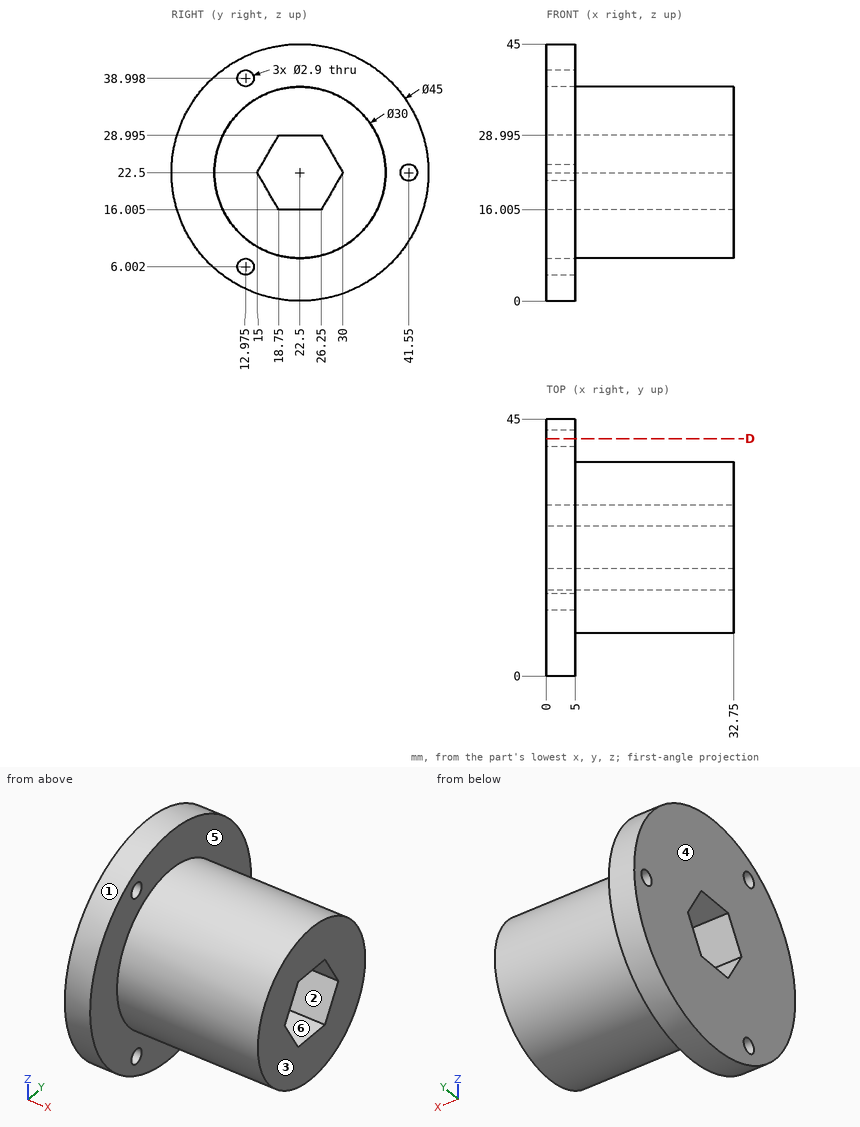
The figure shows three views and two pictorial views of one solid part (mm, origin at its lowest corner). Answer the questions. A direction names the side the tool comes from. Round coordinates to 2 decimals unless told otherwise and drop trailing zeros. Order: outer loops, then holes, each group sorted by start corner. A loop starts at its lowest first (then second) coordinate and runs counter-clockwise, first axis right, second up.
Q1. Find the intervals of material crossed by line 1 along Y through (x, z) = (2.2, 22.5); line 2 along Y through (x, z) = (1, 22) (1 decimal); line 3 along X through (y, z) = (43, 28), in increasing order.
Solution:
line 1: y = 0 to 15, 30 to 40.1, 43 to 45
line 2: y = 0 to 15.3, 29.7 to 40.2, 42.9 to 45
line 3: x = 0 to 5
Q2. The mould has two halves that part along Y. Classify the marked faces 1, 2 and 3: pulls with the +Y half, pulls with the -Y half, needs draft (parallel to the pull), parting line crosses it, or undercut.
Solution:
face 1: parting line crosses it
face 2: undercut
face 3: needs draft
Q3. A tool of negligible diameter and unlimited length cuts with its end or side. For the marked faces 4, 5 and 6, from which of +Z, -Z, +X, -X, +Y, -Y can it reach the whole face along a straight path? Write none if from no direction.
Solution:
face 4: +Z, -Z, -X, +Y, -Y
face 5: +X
face 6: +X, -X
Q4. Given pin 1 Ø1 at (x, z) = (29, 11) entering from +Y; pin 2 Ø6 at (x, y) = (18, 22) entering from -Z; pin 3 Ø1.5 at (x, y) = (16, 33.5) entering from -Z, each flat-ended and moving along its own axis, determine where each tip first touches the part or whether it passes through.
Solution:
pin 1: stops at y = 32.7
pin 2: stops at z = 7.5
pin 3: stops at z = 11.55
Q5. A cutting plane is placed at D-D, the plane y = 41.55. Determine the outline of the cut face in (x, z), then the cut area to 3 significant figures.
Solution:
outline: (0, 10.53) - (5, 10.53) - (5, 21.05) - (0, 21.05) - close; (0, 23.95) - (5, 23.95) - (5, 34.47) - (0, 34.47) - close
area: 105 mm2
